Can you work these out from the model? Positions are in its coordinate system, mm. A direction names the side the tool comes from. Give positions to 0.01 mm unless a question says otherwise; leave off trailing zeros. Order: outer loops, then holes, each group sorted by start corner. A loop starts at its lowest first (then second) coordinate and runs counter-clockwise, first axis right, second up. Notation, with made-up numbers: (89, 8) - (118, 8) arc R14 cw to (118, 17) - close; hole circle Ø6 at (36.25, -17.75). An arc over 180 degrees is marked (long way). Use one line per item in the form item = value. Start each with the question number.
1) We'd pull the mould along Y, two halves only. Please class faces 1 (the flat face through (39, -13.711, 15)), 2 (the flat face through (40, -38, 4)), 3 (the cylindrical face through (38.35, -47.76, 4.93)), 4 (the flat face through (33, -48.83, 5)): released by +Y, released by -Y, zero draft, split by the parting line, or undercut.
2) Suppose I cut it at B-B, the plane y = -58.5. Write out the boundary of the cut face in (x, z).
3) For pin 1 (7 mm diameter, centred on x = 5, y = -58.5, fed in from +Z); pin 2 (7 mm diameter, centred on y = -56.5, z = 10.5, fed in from -X); pin 3 (5.5 mm diameter, centred on x = 33, z = 4.5, fed in from -Y); pin 4 (21 mm diameter, centred on x = 24.5, y = -31.5, fed in from +Z), each with a flat end and sliding along its axis, tell me the tip position at first contact or that it passes through.
4) Which directions (+Z, -Z, +X, -X, +Y, -Y) give clear straight access to the entire face, cutting with the end or side of a thin tool? Please do faces 5 (the flat face through (66.06, -51.29, 11.67)), 6 (the flat face through (66, -49.789, 15)), 7 (the cylindrical face through (79, -5, 14)), 8 (the cylindrical face through (34.61, -50.86, 3.66)).
5) Suppose I cut it at D-D, the plane y = -37. Write out the boundary of the cut face in (x, z), and give its area (3 significant figures).
6) Please list where these lines run through material, in increasing order: probe 1 along Y at (x, z) = (75, 8); probe 2 along X at (y, z) = (-36, 3.5); probe 3 along Z at (x, y) = (40, -46).
7) Suppose I cut it at C-C, the plane x = 23. Write out the boundary of the cut face in (y, z).
8) Suppose I cut it at A-A, the plane x = 75. Write out the boundary of the cut face in (y, z), and give its area (3 significant figures).
```python
from build123d import *
from OCP.BRepFilletAPI import BRepFilletAPI_MakeChamfer

# Parameters (mm, degrees)
SKETCH_1_W                  = 80
SKETCH_1_H                  = 63.5
EXTRUDE_1_DEPTH             = 16
CUT_EXTRUDE_1_DEPTH         = 104.383992958
SKETCH_15_W                 = 25
SKETCH_15_H                 = 14.711451884
CUT_EXTRUDE_4_DEPTH         = 7
SKETCH_16_W                 = 25
SKETCH_16_H                 = 10.67
CUT_EXTRUDE_5_DEPTH         = 9
SKETCH_17_R                 = 2.5
CUT_EXTRUDE_6_DEPTH         = 4
M4X0_72_D                   = 3.3
M4X0_72_DEPTH               = 10
M4X0_72_TIP                 = 0.991420021
CUT_EXTRUDE_7_DEPTH         = 4
SKETCH_26_R                 = 3.25
CUT_EXTRUDE_8_DEPTH         = 38
HOLE_WIZARD_M41_D           = 4.5
HOLE_WIZARD_M41_CBORE_D     = 8
HOLE_WIZARD_M41_CBORE_DEPTH = 4
CHAMFER_2_SIZE              = 1
CHAMFER_2_SIZE2             = 2


with BuildPart() as part:
    # Эскиз1 → Бобышка-Вытянуть1 (new body)
    with BuildSketch(Plane.XY):
        with Locations((40, -31.75)):
            Rectangle(SKETCH_1_W, SKETCH_1_H)
    extrude(amount=EXTRUDE_1_DEPTH)

    # Эскиз2 → Вырез-Вытянуть1 (cut, through all)
    with BuildSketch(Plane.ZY):
        Polygon((9, -10.67), (16, -14.711451884), (16, -48.788548116), (9, -52.83), align=None)
    extrude(amount=-CUT_EXTRUDE_1_DEPTH, mode=Mode.SUBTRACT)

    # Эскиз15 → Вырез-Вытянуть4 (cut)
    with BuildSketch(Plane.XY.offset(16)):
        with Locations((40, -56.144274058)):
            Rectangle(SKETCH_15_W, SKETCH_15_H)
    extrude(amount=-CUT_EXTRUDE_4_DEPTH, mode=Mode.SUBTRACT)

    # Эскиз16 → Вырез-Вытянуть5 (cut)
    with BuildSketch(Plane.XY.offset(9)):
        with Locations((40, -58.165)):
            Rectangle(SKETCH_16_W, SKETCH_16_H)
    extrude(amount=-CUT_EXTRUDE_5_DEPTH, mode=Mode.SUBTRACT)

    # Эскиз17 → Вырез-Вытянуть6 (cut)
    with BuildSketch(Plane.XZ.offset(52.83)):
        with Locations(Location((32.5, 5, 0), (0, 0, 270))):
            Circle(SKETCH_17_R)
        with Locations(Location((47.5, 5, 0), (0, 0, 90))):
            Circle(SKETCH_17_R)
    extrude(amount=-CUT_EXTRUDE_6_DEPTH, mode=Mode.SUBTRACT)

    # Отверстие обработанное метчиком M4x0.72
    with Locations(Plane(origin=(0, -52.83, 0), x_dir=(-1, 0, 0), z_dir=(0, -1, 0))):
        with Locations((-40, -5)):
            Hole(M4X0_72_D / 2, depth=M4X0_72_DEPTH)
            with Locations((0, 0, -(M4X0_72_DEPTH + M4X0_72_TIP / 2))):  # 118° drill point
                Cone(0, M4X0_72_D / 2, M4X0_72_TIP, mode=Mode.SUBTRACT)

    # Эскиз25 → Вырез-Вытянуть7 (cut)
    with BuildSketch(Plane.XY.offset(9)):
        with BuildLine():
            Line((43.1, -18.711451884), (43.1, -25.711451884))
            ThreePointArc((43.1, -25.711451884), (40, -28.811451884), (36.9, -25.711451884))
            Line((36.9, -25.711451884), (36.9, -18.711451884))
            ThreePointArc((36.9, -18.711451884), (40, -15.611451884), (43.1, -18.711451884))
        make_face()
    extrude(amount=-CUT_EXTRUDE_7_DEPTH, mode=Mode.SUBTRACT)

    # Эскиз26 → Вырез-Вытянуть8 (cut)
    with BuildSketch(Plane(origin=(0, 0, 0), x_dir=(1, 0, 0), z_dir=(0, 1, 0))):
        with Locations(Location((40, -4.5, 0), (0, 0, 270))):
            Circle(SKETCH_26_R)
    extrude(amount=-CUT_EXTRUDE_8_DEPTH, mode=Mode.SUBTRACT)

    # Цековка для винта с внутренним шестигранником M41 (through all)
    with Locations(Plane(origin=(30.759227947, 26.793365177, 16), x_dir=(-1, 0, 0), z_dir=(0, 0, 1))):
        with Locations((-44.240772053, 31.793365177), (-44.240772053, 85.293365177), (25.759227947, 85.293365177), (25.759227947, 31.793365177)):
            CounterBoreHole(HOLE_WIZARD_M41_D / 2, HOLE_WIZARD_M41_CBORE_D / 2, HOLE_WIZARD_M41_CBORE_DEPTH)

    # Фаска2: one chamfer whose edges measure the first distance from different faces: ONE call of the kernel's chamfer builder (chamfer() names one face for all edges)
    chamfer_2_edges_1 = [part.edges().sort_by_distance(p)[0] for p in [
        (40, -14.711451884, 16),
    ]]
    chamfer_2_side_1 = [part.faces().sort_by_distance(p)[0] for p in [
        (40, -7.575743279, 16),
    ]]
    chamfer_2_edges_2 = [part.edges().sort_by_distance(p)[0] for p in [
        (66.25, -48.788548116, 16),
    ]]
    chamfer_2_side_2 = [part.faces().sort_by_distance(p)[0] for p in [
        (65.008612302, -55.810060435, 16),
    ]]
    chamfer_2_edges_3 = [part.edges().sort_by_distance(p)[0] for p in [
        (13.75, -48.788548116, 16),
    ]]
    chamfer_2_side_3 = [part.faces().sort_by_distance(p)[0] for p in [
        (14.991387698, -55.810060435, 16),
    ]]
    chamfer_2 = BRepFilletAPI_MakeChamfer(part.part.solid().wrapped)
    for e in chamfer_2_edges_1:
        chamfer_2.Add(CHAMFER_2_SIZE, CHAMFER_2_SIZE2, e.wrapped, chamfer_2_side_1[0].wrapped)  # the first distance lies on this face
    for e in chamfer_2_edges_2:
        chamfer_2.Add(CHAMFER_2_SIZE, CHAMFER_2_SIZE2, e.wrapped, chamfer_2_side_2[0].wrapped)  # the first distance lies on this face
    for e in chamfer_2_edges_3:
        chamfer_2.Add(CHAMFER_2_SIZE, CHAMFER_2_SIZE2, e.wrapped, chamfer_2_side_3[0].wrapped)  # the first distance lies on this face
    add(Compound.cast(chamfer_2.Shape()), mode=Mode.REPLACE)


solid = part.part
```
Result sheet:
q1.face_1 = undercut
q1.face_2 = released by +Y
q1.face_3 = zero draft
q1.face_4 = released by -Y
q2.outline = (0, 0) - (2.75, 0) - (2.75, 12) - (1, 12) - (1, 16) - (0, 16) - close; (7.25, 0) - (27.5, 0) - (27.5, 16) - (9, 16) - (9, 12) - (7.25, 12) - close; (52.5, 0) - (72.75, 0) - (72.75, 12) - (71, 12) - (71, 16) - (52.5, 16) - close; (77.25, 0) - (80, 0) - (80, 16) - (79, 16) - (79, 12) - (77.25, 12) - close
q3.pin_1 = 12
q3.pin_2 = 0
q3.pin_3 = -52.83
q3.pin_4 = 9
q4.face_5 = +X, -X
q4.face_6 = +Z, +X, -X
q4.face_7 = +Z
q4.face_8 = -Y
q5.outline = (0, 0) - (80, 0) - (80, 9) - (0, 9) - close; hole circle Ø6.5 at (40, 4.5)
q5.area = 687 mm²
q6.probe_1 = -63.5 to -60.75, -56.25 to -7.25, -2.75 to 0
q6.probe_2 = 0 to 36.91, 43.09 to 80
q6.probe_3 = 0 to 3.35, 6.65 to 9
q7.outline = (-63.5, 0) - (0, 0) - (0, 16) - (-13.71, 16) - (-13.71, 14.27) - (-10.67, 9) - (-52.83, 9) - (-49.79, 14.27) - (-49.79, 16) - (-63.5, 16) - close
q8.outline = (-63.5, 0) - (-60.75, 0) - (-60.75, 12) - (-62.5, 12) - (-62.5, 16) - (-63.5, 16) - close; (-56.25, 0) - (-7.25, 0) - (-7.25, 12) - (-9, 12) - (-9, 16) - (-13.71, 16) - (-13.71, 14.27) - (-10.67, 9) - (-52.83, 9) - (-49.79, 14.27) - (-49.79, 16) - (-54.5, 16) - (-54.5, 12) - (-56.25, 12) - close; (-2.75, 0) - (0, 0) - (0, 16) - (-1, 16) - (-1, 12) - (-2.75, 12) - close
q8.area = 575 mm²
